Read the model definition and answer for the solid it produces. Units are mm, in the model's axes. A direction names the side the tool comes from. Give positions to 0.01 mm unless a question says otherwise; leave off trailing zeros. Write each loop counter-clockwise with the first axis right and the second up, starting at its lowest first coordinate (ties: lowest second). Pieces come first, ordered by that corner, then holes. Notation, with made-up numbers: (50.25, -16) - (108.25, -16) arc R15 ccw to (108.25, 7) - close; hole circle Ø1 at (88.25, 40). An arc over 180 degrees is marked (long way). Answer as CSV lines item,"result".
```python
from build123d import *

# Parameters (mm, degrees)
SKETCH1_R           = 30
BOSS_EXTRUDE1_DEPTH = 5
SKETCH2_R           = 10
BOSS_EXTRUDE2_DEPTH = 90
SKETCH4_R           = 6
CUT_EXTRUDE2_DEPTH  = 200
SKETCH5_R           = 1.5
CUT_EXTRUDE3_DEPTH  = 10
SKETCH6_R           = 8
CUT_EXTRUDE4_DEPTH  = 10
SKETCH8_R           = 2
CUT_EXTRUDE5_DEPTH  = 20
CUT_EXTRUDE6_START  = -70
SKETCH10_R          = 10
CUT_EXTRUDE6_DEPTH  = 70
SKETCH12_R          = 8.1
CUT_EXTRUDE7_DEPTH  = 10
SKETCH13_R          = 2
CUT_EXTRUDE8_DEPTH  = 20


with BuildPart() as part:
    # Sketch1 → Boss-Extrude1 (new body)
    with BuildSketch(Plane(origin=(0, 0, 0), x_dir=(1, 0, 0), z_dir=(0, 1, 0))):
        with Locations(Location((0, 0, 0), (0, 0, 270))):
            Circle(SKETCH1_R)
    extrude(amount=BOSS_EXTRUDE1_DEPTH)

    # Sketch2 → Boss-Extrude2 (add)
    with BuildSketch(Plane(origin=(0, 5, 0), x_dir=(1, 0, 0), z_dir=(0, 1, 0))):
        with Locations(Location((0, 0, 0), (0, 0, 90))):
            Circle(SKETCH2_R)
    extrude(amount=BOSS_EXTRUDE2_DEPTH)

    # Sketch4 → Cut-Extrude2 (cut)
    with BuildSketch(Plane(origin=(0, 95, 0), x_dir=(1, 0, 0), z_dir=(0, 1, 0))):
        with Locations(Location((0, 0, 0), (0, 0, 270))):
            Circle(SKETCH4_R)
    extrude(amount=-CUT_EXTRUDE2_DEPTH, mode=Mode.SUBTRACT)

    # Sketch5 → Cut-Extrude3 (cut)
    with BuildSketch(Plane(origin=(0, 5, 0), x_dir=(1, 0, 0), z_dir=(0, 1, 0))):
        with Locations(Location((0, 14.969819474, 0), (0, 0, 270))):
            Circle(SKETCH5_R)
        with Locations(Location((14.969819474, 0, 0), (0, 0, 270))):
            Circle(SKETCH5_R)
        with Locations(Location((0, -14.969819474, 0), (0, 0, 270))):
            Circle(SKETCH5_R)
        with Locations(Location((-14.969819474, 0, 0), (0, 0, 270))):
            Circle(SKETCH5_R)
    extrude(amount=-CUT_EXTRUDE3_DEPTH, mode=Mode.SUBTRACT)

    # Sketch6 → Cut-Extrude4 (cut)
    with BuildSketch(Plane(origin=(0, 95, 0), x_dir=(1, 0, 0), z_dir=(0, 1, 0))):
        with Locations(Location((0, 0, 0), (0, 0, 270))):
            Circle(SKETCH6_R)
    extrude(amount=-CUT_EXTRUDE4_DEPTH, mode=Mode.SUBTRACT)

    # Sketch8 → Cut-Extrude5 (cut)
    with BuildSketch(Plane(origin=(0, 95, -10), x_dir=(-1, 0, 0), z_dir=(0, 0, -1))):
        with Locations((0, -5)):
            Circle(SKETCH8_R)
    extrude(amount=-CUT_EXTRUDE5_DEPTH, mode=Mode.SUBTRACT)

    # Sketch10 → Cut-Extrude6 (cut)
    with BuildSketch(Plane(origin=(0, 95, 0), x_dir=(1, 0, 0), z_dir=(0, 1, 0)).offset(CUT_EXTRUDE6_START)):
        with Locations(Location((0, 0, 0), (0, 0, 90))):
            Circle(SKETCH10_R)
    extrude(amount=CUT_EXTRUDE6_DEPTH, mode=Mode.SUBTRACT)

    # Sketch12 → Cut-Extrude7 (cut)
    with BuildSketch(Plane(origin=(0, 25, 0), x_dir=(1, 0, 0), z_dir=(0, 1, 0))):
        with Locations(Location((0, 0, 0), (0, 0, 270))):
            Circle(SKETCH12_R)
    extrude(amount=-CUT_EXTRUDE7_DEPTH, mode=Mode.SUBTRACT)

    # Sketch13 → Cut-Extrude8 (cut)
    with BuildSketch(Plane(origin=(0, 95, -10), x_dir=(-1, 0, 0), z_dir=(0, 0, -1))):
        with Locations((0, -75)):
            Circle(SKETCH13_R)
    extrude(amount=-CUT_EXTRUDE8_DEPTH, mode=Mode.SUBTRACT)


solid = part.part
```
(1) The mould has two halves that part along X. Classify faces 1 (the flat face through (0, 5, 13)), 2 (the cylindrical face through (1.32, 2.46, -29.97)), 3 (the cylindrical face through (0, 22, -9)), 4 (the cylindrical face through (1.6, 18.8, 8.9)): +X half, -X half, draft (parallel to the pull), parting line (faces both ways), or undercut.
Worked out:
face 1,"draft"
face 2,"parting line"
face 3,"undercut"
face 4,"undercut"
(2) A cutting plane is placed at A-A (z = 0). Write down the section's boundary in (x, y), and give its area (3 significant figures).
Worked out:
outline,"(-30, 0) - (-16.47, 0) - (-16.47, 5) - (-30, 5) - close; (-13.47, 0) - (-6, 0) - (-6, 15) - (-8.1, 15) - (-8.1, 25) - (-10, 25) - (-10, 5) - (-13.47, 5) - close; (6, 0) - (13.47, 0) - (13.47, 5) - (10, 5) - (10, 25) - (8.1, 25) - (8.1, 15) - (6, 15) - close; (16.47, 0) - (30, 0) - (30, 5) - (16.47, 5) - close"
area,"328 mm^2"
(3) For faces 5 (the cylindrical face through (-3, 14.86, -9.54)), 6 (the cylindrical face through (1.802, 7.605, 5.723)), determine the directions among +Z, -Z, +X, -X, +Y, -Y from which every point of the face is accessible in a straight line to the end or side of a thin tool.
Worked out:
face 5,"+Y"
face 6,"+Y, -Y"
(4) Find the intervals of material crossed by L1, parallel to X at y = 1.95, z = 0; L2, parallel to Y at x = 11, z = -23; L3, parallel to Y at x = -6, z = -3.5, in increasing order.
Worked out:
L1,"x = -30 to -16.47, -13.47 to -6, 6 to 13.47, 16.47 to 30"
L2,"y = 0 to 5"
L3,"y = 0 to 15"
(5) A cutting plane is placed at C-C (y = 20). Write down the section's boundary in (x, z).
Worked out:
outline,"(-2, -9.8) - (-2, -7.85) arc R8.1 cw to (-2, 7.85) - (-2, 9.8) arc R10 ccw to start; (2, -9.8) arc R10 ccw to (2, 9.8) - (2, 7.85) arc R8.1 cw to (2, -7.85) - close"
(6) A cutting plane is placed at B-B (x = 0). Count the separate pieces of the cut face and the enclosed holes in it, and give its area (3 significant figures).
Worked out:
separate pieces,"6"
enclosed holes,"0"
area,"313 mm^2"
(7) A cutting plane is placed at D-D (z = 18). Write down the section's boundary in (x, y), and give its area (3 significant figures).
Worked out:
outline,"(-24, 0) - (24, 0) - (24, 5) - (-24, 5) - close"
area,"240 mm^2"
(8) Each of these flat-tipped pins is pushed along its axis until it touches: P1, Ø1.5, axis at x = 11, y = 5, coming from the -Z side; P2, Ø9.5, axis at x = 0, z = 0, coming from the +Y side; P3, Ø3.5, axis at x = 14.97, z = 0, coming from the +Y side; P4, Ø4, axis at x = -2, y = 18, coming from the -Z side. Where does it stop, or does it pass through?
Worked out:
P1,"stops at z = -28.19"
P2,"passes through"
P3,"stops at y = 5"
P4,"stops at z = -10"
